Verification items for the finished model (mm, model axes). Round coordinates to 2 decimals unless told otherwise and drop trailing zeros. Write each loop counter-clockwise with the first axis right and the second up, starting at its lowest first coordinate (ties: lowest second). Pieces come first, ordered by that corner, then holes.
from build123d import *

# Parameters (mm, degrees)
MODEL_R         = 2.35
MODEL_W         = 10
MODEL_H         = 2.3
MODEL_H_2       = 2.20013503
EXTRUDE_1_DEPTH = 1


with BuildPart() as part:
    # Model → 凸台-拉伸1 (new body)
    with BuildSketch(Plane.XY):
        Polygon((3.002178354, 2.656404454), (33.252178354, 2.656404454), (52.002178354, 2.656404454), (52.002178354, 32.582558285), (50.002178354, 32.582558285), (50.002178354, 62.582558285), (52.002178354, 62.582558285), (52.002178354, 92.582558285), (40.002178354, 92.582558285), (40.002178354, 90.382558285), (30.002178354, 90.382558285), (30.002178354, 92.582558285), (25.002178354, 92.582558285), (25.002178354, 90.382558285), (15.002178354, 90.382558285), (15.002178354, 92.582558285), (3.002178354, 92.582558285), (3.002178354, 62.582558285), (5.002178354, 62.582558285), (5.002178354, 32.582558285), (3.002178354, 32.582558285), align=None)
        with Locations((27.502178354, 42.933185696)):
            Circle(MODEL_R, mode=Mode.SUBTRACT)
        with Locations((20.002178354, 46.632557075)):
            Rectangle(MODEL_W, MODEL_H, mode=Mode.SUBTRACT)
        with Locations((20.002178354, 14.429981905)):
            Rectangle(MODEL_W, MODEL_H_2, mode=Mode.SUBTRACT)
        with Locations((35.002178354, 14.429981905)):
            Rectangle(MODEL_W, MODEL_H_2, mode=Mode.SUBTRACT)
        with Locations((35.002178354, 46.632557075)):
            Rectangle(MODEL_W, MODEL_H, mode=Mode.SUBTRACT)
    extrude(amount=EXTRUDE_1_DEPTH)


solid = part.part
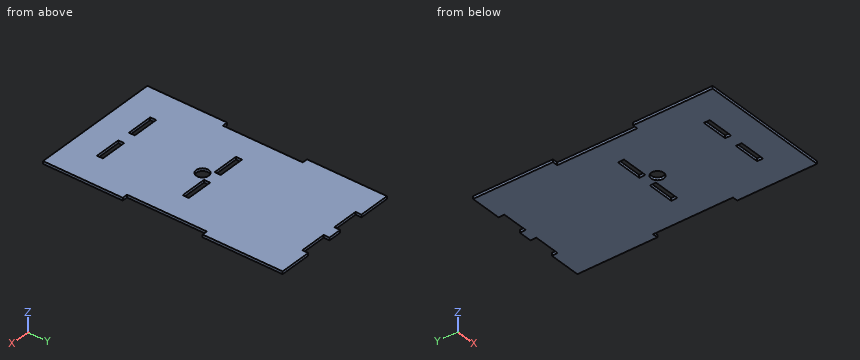
Q1. Depth check by flat-ended pin: P1, Ø1, axis at x = 43.5, y = 50.5, coming from the -Z side; P2, Ø4, axis at x = 27.5, y = 42.93, coming from the +Z side; P3, Ø0.5, axis at y = 46.5, z = 0.5, coming from the -X side; P4, Ø0.5, axis at y = 46, z = 0.5, coming from the +X side. Enter the tip coordinate at first touch or a pass-through.
Recorded:
P1: stops at z = 0
P2: passes through
P3: stops at x = 5
P4: stops at x = 50
Q2. Sectioned sample at C-C (z = 0.2). Give the number of separate pieces and of enclosed holes in the cut face, plus the area to 3 significant figures.
Recorded:
separate pieces: 1
enclosed holes: 5
area: 4,140 mm2
Q3. Sectioned sample at A-A (x = 21). Enter the section's corners in (y, z), plus the area to 3 significant figures.
Recorded:
outline: (2.66, 0) - (13.33, 0) - (13.33, 1) - (2.66, 1) - close; (15.53, 0) - (45.48, 0) - (45.48, 1) - (15.53, 1) - close; (47.78, 0) - (90.38, 0) - (90.38, 1) - (47.78, 1) - close
area: 83.2 mm2
Q4. Sectioned sample at B-B (y = 56.5). Enter the section's corners in (x, z), plus the area to 3 significant figures.
Recorded:
outline: (5, 0) - (50, 0) - (50, 1) - (5, 1) - close
area: 45.0 mm2
Q5. Material ranges on line 1 along X through (y, z) = (15.5, 0.6); line 2 along Y through (x, z) = (30.5, 0.7); line 3 along X through (y, z) = (62.5, 0.3), recorded low to high.
Recorded:
line 1: x = 3 to 15, 25 to 30, 40 to 52
line 2: y = 2.66 to 13.33, 15.53 to 45.48, 47.78 to 90.38
line 3: x = 5 to 50
